Geometry check sheet. Reference: drawing and pictorial views, mm from the part's lowest x, y, z. Give positions to 0.01 mm unless a question says otherwise; leave off trailing zeros. Write each loop counter-clockwise with the first axis right and the second up, starting at its lowest first coordinate (ties: lowest second). Pieces come first, ordered by that corner, then holes. Notation, with made-up numbers: (70.25, 24) -> (83.25, 24) arc R17 ccw to (83.25, 51) -> close; hole circle Ø10 at (14.5, 32.25). An arc over 180 degrees is marked (long way). Use a Markdown table: item, result. Add a question column.
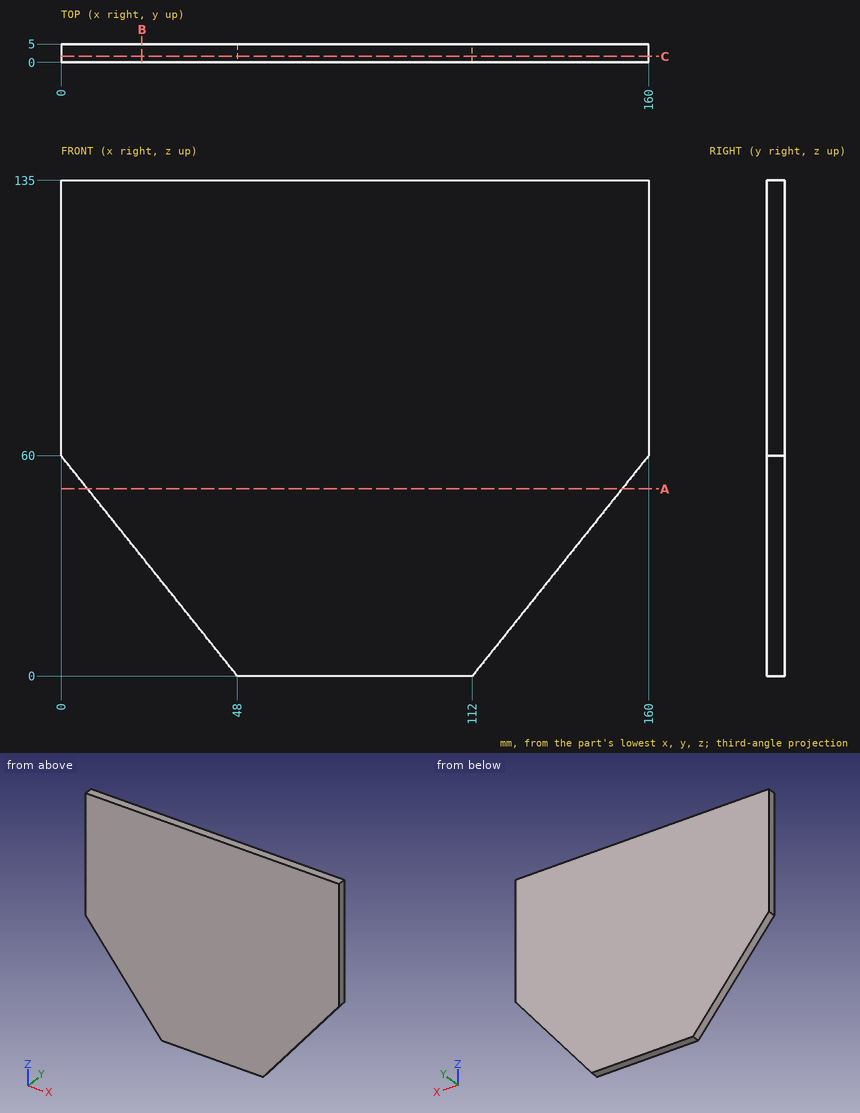
1) Sectioned sample at A-A, the plane z = 51. Enter the section's corners in (x, y).
2) Material ranges on probe 1 along Z at (x, y) = (17, 4.7); probe 2 along Z at (x, y) = (127.5, 1.55) (3 decimals); probe 3 along X at (y, z) = (3.65, 20), recorded low to high. Write a range as [from, to].
3) Gauge pin test, flat ends, axial feed: P1, Ø3, axis at y = 4, z = 43.5, coming from the -X side; P2, Ø1.5, axis at y = 2.5, z = 16.5, coming from the +X side. Record the tip position at first contact, or that the pin passes through.
4) Sectioned sample at C-C, the plane y = 1.65. Enter the section's corners in (x, z), and give its area (3 significant figures).
5) Sectioned sample at B-B, the plane x = 22. Enter the section's corners in (y, z).
Check values:
| question | item | result |
|---|---|---|
| 1 | outline | (7.2, 0) -> (152.8, 0) -> (152.8, 5) -> (7.2, 5) -> close |
| 2 | probe 1 | [38.75, 135] |
| 2 | probe 2 | [19.375, 135] |
| 2 | probe 3 | [32, 128] |
| 3 | P1 | x = 12 |
| 3 | P2 | x = 125.8 |
| 4 | outline | (0, 60) -> (48, 0) -> (112, 0) -> (160, 60) -> (160, 135) -> (0, 135) -> close |
| 4 | area | 18,700 mm² |
| 5 | outline | (0, 32.5) -> (5, 32.5) -> (5, 135) -> (0, 135) -> close |
